The figure shows three views and two pictorial views of one solid part (mm, origin at its lowest corner). Answer the questions. Coordinates: 2 decimals unless noted, no trailing zeros. Loops run counter-clockwise (first coordinate to the right, second up) from the corner with the lowest first, then second, coordinate; pieces in that order, holes last.
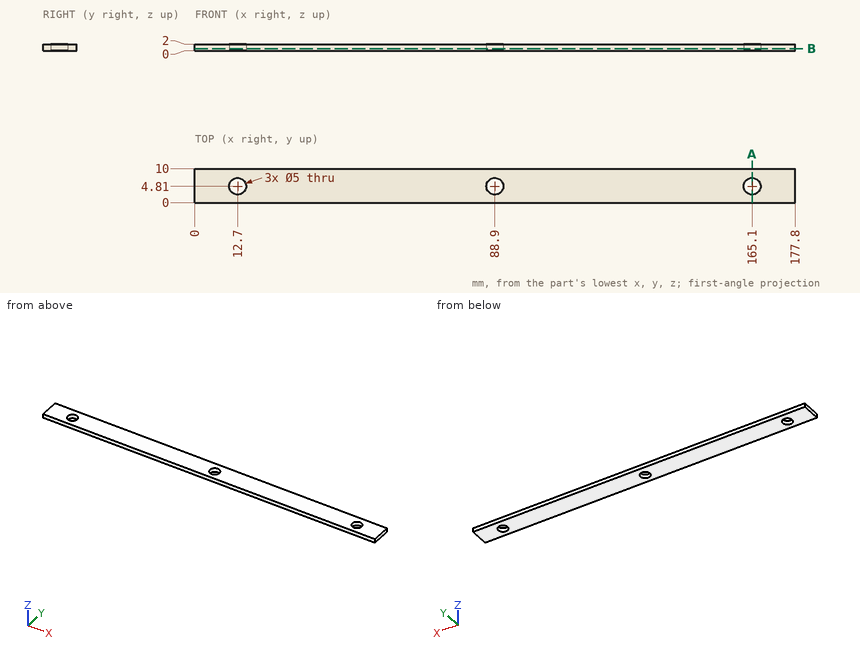
Q1. A cutting plane is placed at A-A (x = 165.1). Give the vertices of the cut face in (y, z), then the cut area to 3 significant figures.
Findings below:
outline: (0, 0) - (2.31, 0) - (2.31, 2) - (0, 2) - close; (7.31, 0) - (10, 0) - (10, 2) - (7.31, 2) - close
area: 10.0 mm2
Q2. Straight lines are drawn through the part: probe 1 along Y at (x, z) = (88.9, 0.9); probe 2 along X at (y, z) = (5.5, 1.9); probe 3 along X at (y, z) = (3.5, 1.75). For each, find the intervals that lie inside material, in ascending order.
Findings below:
probe 1: y = 0 to 2.31, 7.31 to 10
probe 2: x = 0 to 10.3, 15.1 to 86.5, 91.3 to 162.7, 167.5 to 177.8
probe 3: x = 0 to 10.57, 14.83 to 86.77, 91.03 to 162.97, 167.23 to 177.8
Q3. A cutting plane is placed at B-B (z = 0.6). Give the vertices of the cut face in (x, y), then the cut area to 3 significant figures.
Findings below:
outline: (0, 0) - (177.8, 0) - (177.8, 10) - (0, 10) - close; hole circle Ø5 at (12.7, 4.81); hole circle Ø5 at (88.9, 4.81); hole circle Ø5 at (165.1, 4.81)
area: 1,720 mm2
